The model under review builds one solid part; all positions refer to its coordinate system, in mm. Give positions to 0.01 mm unless a question says otherwise; leave off trailing zeros. Loops run counter-clockwise (first coordinate to the right, second up) from the corner with the lowest first, then second, coordinate; pieces in that order, holes last. Notation, with made-up numbers: (68, 62) -> (90, 62) arc R14 cw to (90, 86) -> close; hole circle Ø4 at (17.5, 1.5). An arc over 180 degrees is marked (long way). Write each question's results on one line, items separated by ' | '. Start each with the question number.
Q1. We need section A-A (z = 0). Write out the cut boundary in (x, y), plus the area to 4 significant figures.
Q2. Wall thickness on L1, parallel to Z at x = 1, y = 189; L2, parallel to Y at x = 5, z = 1: over which ranges is each line inside the solid? List them lowest first. Write a range as [from, to].
Q3. Insertion check: pin 1 Ø1 at (y, z) = (158, -0.5) entering from -X; pin 2 Ø1 at (x, y) = (-1, 90.5) entering from -Z; pin 3 Ø1.5 at (y, z) = (55, 1.5) entering from -X. Each pin has a flat end and moves straight along its axis. Give the tip position at first contact, or say it passes through.
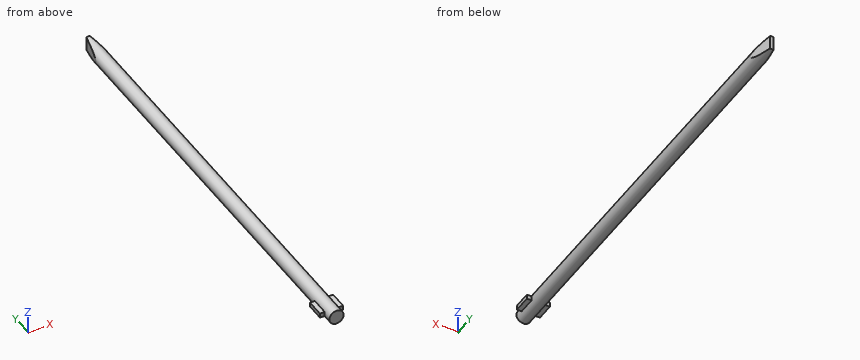
Solid Edge part; units mm, degrees
sketch "Sketch1" plane through (0, 0, 0) normal (0, -1, 0) x (1, 0, 0)
  circle A0 centre (0, 0) radius 4
extrude "Protrusion1" add sketch "Sketch1" against normal blind 250
sketch "Sketch2" plane through (0, 0, 0) normal (0, 0, 1) x (1, 0, 0)
  line L0 (4, 250) -> (4, 235)
  line L1 (4, 235) -> (1, 250)
  line L2 (1, 250) -> (4, 250)
  dimension "D1" = 4
  dimension "D2" = 1
extrude "拉伸除料_1" cut sketch "Sketch2" along normal mid plane 43.1543
mirror "Mirror1" about plane through (0, 0, 0) normal (1, 0, 0) of "拉伸除料_1"
sketch "Sketch3" plane through (0, 0, 0) normal (1, 0, 0) x (0, 1, 0)
  line L0 (15, -1.25) -> (5, -1.25)
  line L1 (5, -1.25) -> (5, 1.25)
  line L2 (5, 1.25) -> (15, 1.25)
  line L3 (15, 1.25) -> (15, -1.25)
extrude "拉伸_2" add sketch "Sketch3" along normal mid plane 13
Output:
1) outline: (-6.5, 5) -> (-4, 5) -> (-4, 0) -> (4, 0) -> (4, 5) -> (6.5, 5) -> (6.5, 15) -> (4, 15) -> (4, 235) -> (1, 250) -> (-1, 250) -> (-4, 235) -> (-4, 15) -> (-6.5, 15) -> close | area: 2,005 mm2
2) L1: [-3.87, 3.87] | L2: [5, 15]
3) pin 1: x = -4 | pin 2: z = -3.97 | pin 3: x = -3.93
